Geometry check sheet. Reference: the model listing, model coordinates, mm. A direction names the side the tool comes from. Give positions to 0.01 mm unless a question says otherwise; leave off trailing zeros. Write each loop counter-clockwise with the first axis right and the second up, starting at its lowest first coordinate (ties: lowest second). Pieces come first, ordered by that corner, then holes. Notation, with made-up numbers: (78.25, 23) -> (119.25, 23) arc R28 ccw to (119.25, 49) -> close; hole circle Ø10 at (-31, 88). An arc over 180 degrees is marked (long way). Use a Markdown table: item, result. Add a question column.
from build123d import *

# Parameters (mm, degrees)
MAIN_DEPTH                         = 10
ESQUISSE4_W                        = 2.9
ESQUISSE4_H                        = 20
MAKERBEAMFIXVERTICAL_DEPTH         = 1
MAKERBEAMVERTICALHOLE_DEPTH        = 31
MAKERBEAMVERTICALHOLE_DEPTH_BACK   = 31
ESQUISSE2_R                        = 1.5
ESQUISSE5_W                        = 20
ESQUISSE5_H                        = 2.9
MAKERBEAMFIXHORIZONTAL_DEPTH       = 1
MAKERBEAMHORIZONTALHOLE_DEPTH      = 31
MAKERBEAMHORIZONTALHOLE_DEPTH_BACK = 31
ESQUISSE3_R                        = 1.5
SKETCH1_R                          = 1.35
WINDOWFIXHOLE_DEPTH                = 31
SKETCH2_W                          = 2.5
SKETCH2_H                          = 20
WINDOW_DEPTH                       = 31


with BuildPart() as part:
    # Esquisse1 → Main (new body)
    with BuildSketch(Plane.XY):
        with BuildLine():
            Line((0, 0), (20, 0))
            Line((20, 0), (20, 7))
            Line((20, 7), (13, 7))
            ThreePointArc((13, 7), (8.757359313, 8.757359313), (7, 13))
            Line((7, 13), (7, 20))
            Line((7, 20), (0, 20))
            Line((0, 20), (0, 0))
        make_face()
    extrude(amount=MAIN_DEPTH)

    # Esquisse4 → MakerBeamFixVertical (add)
    with BuildSketch(Plane.ZY):
        with Locations((5, 10)):
            Rectangle(ESQUISSE4_W, ESQUISSE4_H)
    extrude(amount=MAKERBEAMFIXVERTICAL_DEPTH)

    # Esquisse2 → MakerBeamVerticalHole (cut, two sides: drawn at the far end of the back side and taken through both)
    with BuildSketch(Plane.ZY.offset(-MAKERBEAMVERTICALHOLE_DEPTH_BACK)):
        with Locations(Location((5, 16, 0), (0, 0, 270))):
            Circle(ESQUISSE2_R)
    extrude(amount=MAKERBEAMVERTICALHOLE_DEPTH + MAKERBEAMVERTICALHOLE_DEPTH_BACK, mode=Mode.SUBTRACT)

    # Esquisse5 → MakerBeamFixHorizontal (add)
    with BuildSketch(Plane(origin=(0, 0, 0), x_dir=(-1, 0, 0), z_dir=(0, -1, 0))):
        with Locations((-10, -5)):
            Rectangle(ESQUISSE5_W, ESQUISSE5_H)
    extrude(amount=MAKERBEAMFIXHORIZONTAL_DEPTH)

    # Esquisse3 → MakerBeamHorizontalHole (cut, two sides: drawn at the far end of the back side and taken through both)
    with BuildSketch(Plane.XZ.offset(-MAKERBEAMHORIZONTALHOLE_DEPTH_BACK)):
        with Locations(Location((16, 5, 0), (0, 0, 270))):
            Circle(ESQUISSE3_R)
    extrude(amount=MAKERBEAMHORIZONTALHOLE_DEPTH + MAKERBEAMHORIZONTALHOLE_DEPTH_BACK, mode=Mode.SUBTRACT)

    # Sketch1 → WindowFixHole (cut, through all)
    with BuildSketch(Plane.XY.offset(10)):
        with Locations((7, 7)):
            Circle(SKETCH1_R)
    extrude(amount=-WINDOWFIXHOLE_DEPTH, mode=Mode.SUBTRACT)

    # Sketch2 → Window (cut, through all)
    with BuildSketch(Plane.ZY):
        with Locations((8.75, 10)):
            Rectangle(SKETCH2_W, SKETCH2_H)
    extrude(amount=-WINDOW_DEPTH, mode=Mode.SUBTRACT)


solid = part.part
1) Material ranges on probe 1 along Z at (x, y) = (16, 3.75); probe 2 along X at (y, z) = (2.25, 5), recorded low to high. Write a range as [from, to].
2) Sectioned sample at C-C, the plane y = 6. Enter the section's corners in (x, z), and give its area (3 significant figures).
3) Tool access check on faces 1 (the face through (-0.5, 7.7, 3.55)), 2 (the face through (7, 16, 3)), 3 (the face through (18.2, -0.5, 3.55)), 4 (the face through (0, 10, 7)), 5 (the face through (7.9, -0.5, 6.45)). Record the directions out of +Z, -Z, +X, -X, +Y, -Y that give a thin tool (end or side, any length) a straight path to the whole face; none if there is none.
4) Gauge pin test, flat ends, axial feed: P1, Ø0.8, axis at x = 18, y = -0.5, coming from the +Z side; P2, Ø0.5, axis at y = 13.5, z = 7, coming from the -X side; P3, Ø2, axis at x = 9.5, z = 5.5, coming from the +Y side. Record the tip position at first contact, or that the pin passes through.
5) Sectioned sample at B-B, the plane x = 6.5. Enter the section's corners in (y, z), and give its area (3 significant figures).
6) Sectioned sample at A-A, the plane z = 5.25. Enter the section's corners in (x, y), and give its area (3 significant figures).
7) Draft check along Y on faces 6 (the face through (20, 3, 4)), 7 (the face through (3.056, 14.614, 4.425)), 8 (the face through (-0.5, 0, 5)). Enter one of: +Y half, -Y half, draft (parallel to the pull), parting line (faces both ways), or undercut.
8) Sectioned sample at D-D, the plane y = 16. Enter the section's corners in (x, z).
Check values:
| question | item | result |
|---|---|---|
| 1 | probe 1 | [0, 3.5], [6.5, 7.5] |
| 1 | probe 2 | [-1, 14.5], [17.5, 20] |
| 2 | outline | (-1, 3.55) -> (0, 3.55) -> (0, 0) -> (6.09, 0) -> (6.09, 7.5) -> (0, 7.5) -> (0, 6.45) -> (-1, 6.45) -> close; (7.91, 0) -> (20, 0) -> (20, 7.5) -> (7.91, 7.5) -> close; hole circle Ø3 at (16, 5) |
| 2 | area | 132 mm² |
| 3 | face 1 | -Z, -X, +Y, -Y |
| 3 | face 2 | +Z, -Z, +X, +Y |
| 3 | face 3 | -Z, +X, -X, -Y |
| 3 | face 4 | +Z, -X, +Y, -Y |
| 3 | face 5 | +Z, +X, -X, -Y |
| 4 | P1 | z = 6.45 |
| 4 | P2 | x = 0 |
| 4 | P3 | y = 9.03 |
| 5 | outline | (-1, 3.55) -> (0, 3.55) -> (0, 0) -> (5.75, 0) -> (5.75, 7.5) -> (0, 7.5) -> (0, 6.45) -> (-1, 6.45) -> close; (8.25, 0) -> (20, 0) -> (20, 7.5) -> (8.25, 7.5) -> close; hole circle Ø3 at (16, 5) |
| 5 | area | 127 mm² |
| 6 | outline | (-1, 0) -> (0, 0) -> (0, -1) -> (14.52, -1) -> (14.52, 7) -> (13, 7) arc R6 cw to (7, 13) -> (7, 14.52) -> (-1, 14.52) -> close; (-1, 17.48) -> (7, 17.48) -> (7, 20) -> (-1, 20) -> close; (17.48, -1) -> (20, -1) -> (20, 7) -> (17.48, 7) -> close; hole circle Ø2.7 at (7, 7) |
| 6 | area | 226 mm² |
| 7 | face 6 | draft |
| 7 | face 7 | undercut |
| 7 | face 8 | -Y half |
| 8 | outline | (0, 0) -> (7, 0) -> (7, 3.5) -> (0, 3.5) -> close; (0, 6.5) -> (7, 6.5) -> (7, 7.5) -> (0, 7.5) -> close |
